from build123d import *

# Parameters (mm, degrees)
BOX013_W          = 14
BOX013_H          = 4.3
BOX013_DEPTH      = 10
CYLINDER021_R     = 28
CYLINDER021_DEPTH = 4
CYLINDER019_R     = 34
CYLINDER019_DEPTH = 13
CYLINDER020_R     = 25
CYLINDER020_DEPTH = 13
TUBE_R            = 34
TUBE_R_2          = 31
TUBE_DEPTH        = 23
EXTRUDE001_DEPTH  = 14
BOX012_W          = 10
BOX012_H          = 6
BOX012_DEPTH      = 10


with BuildPart() as cube013:
    # Box013 → Box013 (new body)
    with BuildSketch(Plane(origin=(64, 38.5, 50.5), x_dir=(1, 0, 0), z_dir=(0, 0, 1))):
        with Locations((7, 2.15)):
            Rectangle(BOX013_W, BOX013_H)
    extrude(amount=BOX013_DEPTH)


with BuildPart() as cylinder021:
    # Cylinder021 → Cylinder021 (new body)
    with BuildSketch(Plane(origin=(40, 40.65, 54), x_dir=(1, 0, 0), z_dir=(0, 0, 1))):
        Circle(CYLINDER021_R)
    extrude(amount=CYLINDER021_DEPTH)


with BuildPart() as cone:
    # Cone → Cone (revolve)
    with BuildSketch(Plane(origin=(40, 40.65, 53), x_dir=(1, 0, 0), z_dir=(0, -1, 0))):
        Polygon((0, 0), (26.5, 0), (31, 14), (0, 14), align=None)
    revolve(axis=Axis((40, 40.65, 53), (0, 0, 1)))


with BuildPart() as cylinder019:
    # Cylinder019 → Cylinder019 (new body)
    with BuildSketch(Plane(origin=(40, 40.65, 54), x_dir=(1, 0, 0), z_dir=(0, 0, 1))):
        Circle(CYLINDER019_R)
    extrude(amount=CYLINDER019_DEPTH)


with BuildPart() as cylinder020:
    # Cylinder020 → Cylinder020 (new body)
    with BuildSketch(Plane(origin=(40, 39.2, 54), x_dir=(1, 0, 0), z_dir=(0, 0, 1))):
        Circle(CYLINDER020_R)
    extrude(amount=CYLINDER020_DEPTH)


with BuildPart() as cut016:
    # Tube → Tube (new body)
    with BuildSketch(Plane(origin=(40, 40.65, 54), x_dir=(1, 0, 0), z_dir=(0, 0, 1))):
        Circle(TUBE_R)
        Circle(TUBE_R_2, mode=Mode.SUBTRACT)
    extrude(amount=TUBE_DEPTH)

    # Fusion010: union Cylinder019, Cylinder020
    add(cylinder019.part)
    add(cylinder020.part)

    # Cut015: cut Cone
    add(cone.part, mode=Mode.SUBTRACT)

    # Cut016: cut Cylinder021
    add(cylinder021.part, mode=Mode.SUBTRACT)


with BuildPart() as extrude001:
    # Sketch001 → Extrude001 (new body)
    with BuildSketch(Plane(origin=(0, 5, 65), x_dir=(1, 0, 0), z_dir=(0, 0, 1))):
        with BuildLine():
            ThreePointArc((16.057001, 41.301956), (16.937891, 38.759239), (19.112253, 37.173829))
            Line((19.112253, 37.173829), (24.78314, 35.869707))
            ThreePointArc((24.78314, 32.174329), (26.017604, 34.022018), (24.78314, 35.869707))
            Line((19.112253, 31.152458), (24.78314, 32.174329))
            ThreePointArc((19.112253, 31.152458), (16.911676, 29.555757), (16.032372, 26.983051))
            Line((15.813344, 26.918672), (16.032372, 26.983051))
            ThreePointArc((15.808908, 41.376289), (14.743203, 34.147153), (15.813344, 26.918672))
            Line((16.057001, 41.301956), (15.808908, 41.376289))
        make_face()
    extrude(amount=EXTRUDE001_DEPTH)


with BuildPart() as extrude001_1:
    # Extrude001 placement: moved
    add(extrude001.part.moved(Location((0, 0, 7))))


with BuildPart() as lid:
    # Box012 → Box012 (new body)
    with BuildSketch(Plane(origin=(7, 36.17, 76), x_dir=(1, 0, 0), z_dir=(0, 0, 1))):
        with Locations((5, 3)):
            Rectangle(BOX012_W, BOX012_H)
    extrude(amount=BOX012_DEPTH)

    # Fusion006: union Extrude001
    add(extrude001_1.part)


with BuildPart() as lid_1:
    # Fusion006 placement: moved
    add(lid.part.moved(Location((0, 1.5, -19))))

    # Fusion024: union Cut016
    add(cut016.part)

    # Cut017: cut Cube013
    add(cube013.part, mode=Mode.SUBTRACT)


solid = lid_1.part
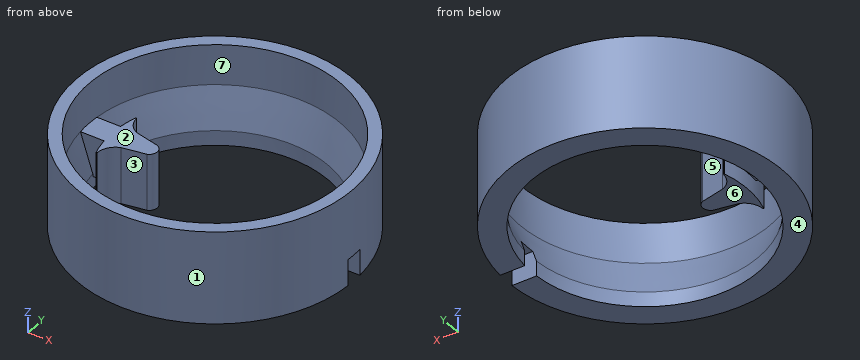
The listing builds one solid part. Answer for the finished solid, in the listing's coordinates (mm). Face numbers are marked on the shaded views. A direction names the side the tool comes from. Give positions to 0.01 mm unless a question says otherwise; leave off trailing zeros. Order: outer loops, then holes, each group sorted by start corner. A loop starts at its lowest first (then second) coordinate and runs counter-clockwise, first axis right, second up. Notation, with made-up numbers: (81, 29.5) -> (103, 29.5) arc R27 ccw to (103, 56.5) -> close; hole circle Ø1 at (70, -28.5). An arc over 180 degrees is marked (long way). Put each result on its own line as item: value.
Item 1: Given P1, Ø6.5, axis at x = 71.5, z = 56, coming from the +Y side; P2, Ø1, axis at x = 16, y = 34, coming from the +Z side; P3, Ø2, axis at x = 71.5, y = 40, coming from the -Z side; P4, Ø12, axis at x = 35, y = 21, coming from the -Z side (1 decimal), each flat-ended and moving along its own axis, determine where each tip first touches the part or whether it passes through.
Established:
P1: stops at y = 59.57
P2: stops at z = 67
P3: stops at z = 60.5
P4: passes through
Item 2: A cutting plane is placed at C-C on y = 40.65. Give the vertices of the cut face in (x, z), plus the area to 3 significant figures.
Established:
outline: (6, 54) -> (12, 54) -> (12, 57) -> (14.74, 57) -> (14.74, 53) -> (26.01, 53) -> (26.01, 67) -> (9, 67) -> (9, 77) -> (6, 77) -> close; (68.91, 60.5) -> (74, 60.5) -> (74, 77) -> (71, 77) -> (71, 67) -> close
area: 350 mm^2
Item 3: A cutting plane is placed at B-B on x = 40. Give the vertices of the cut face in (y, z), plus the area to 3 significant figures.
Established:
outline: (6.65, 54) -> (12.65, 54) -> (12.65, 57.67) -> (9.65, 67) -> (9.65, 77) -> (6.65, 77) -> close; (68.65, 54) -> (74.65, 54) -> (74.65, 77) -> (71.65, 77) -> (71.65, 67) -> (68.65, 57.67) -> close
area: 188 mm^2
Item 4: A cutting plane is placed at D-D on z = 59.5. Give the vertices of the cut face in (x, y) (3 decimals).
Established:
outline: (11.566, 37.67) -> (14.922, 37.67) arc R25 ccw to (15.813, 33.419) -> (16.032, 33.483) arc R4.5 cw to (19.112, 37.652) -> (24.783, 38.674) arc R2 ccw to (24.783, 42.37) -> (19.112, 43.674) arc R4.5 cw to (16.057, 47.802) -> (15.809, 47.876) arc R25 ccw to (14.926, 43.67) -> (11.571, 43.67) arc R28.589 cw to (68.508, 42.8) -> (73.932, 42.8) arc R34 ccw (long way) to (73.932, 38.5) -> (68.508, 38.5) arc R28.589 cw to start
Item 5: Straight lines are drawn through the part: line 1 (Y direction, x = 40, z = 71); line 2 (Y direction, x = 16, z = 61); line 3 (X direction, y = 44.5, z = 71.5). For each, find the intervals that lie inside material, in ascending order.
Established:
line 1: y = 6.65 to 9.65, 71.65 to 74.65
line 2: y = 16.57 to 24.24, 33.47 to 47.82, 57.06 to 64.73
line 3: x = 6.22 to 9.24, 70.76 to 73.78
Item 6: A cutting plane is placed at A-A on z = 55.25. Give the vertices of the cut face in (x, y) (3 decimals).
Established:
outline: (15.809, 47.876) arc R25 ccw to (15.813, 33.419) -> (16.032, 33.483) arc R4.5 cw to (19.112, 37.652) -> (24.783, 38.674) arc R2 ccw to (24.783, 42.37) -> (19.112, 43.674) arc R4.5 cw to (16.057, 47.802) -> close; (67.917, 38.5) arc R28 cw (long way) to (67.917, 42.8) -> (73.932, 42.8) arc R34 ccw (long way) to (73.932, 38.5) -> close
Item 7: For a pull along X with two mould halves and no side action, classify the marked faces 1, 2, 3 and 4 as released by +X, released by -X, zero draft, split by the parting line, or undercut.
Established:
face 1: split by the parting line
face 2: undercut
face 3: undercut
face 4: zero draft
Item 8: For the marked faces 5, 6 and 7, determine the directions among +Z, -Z, +X, -X, +Y, -Y from which every point of the face is accessible in a straight line to the end or side of a thin tool.
Established:
face 5: +Z, -Z
face 6: -Z, +X, -X, +Y, -Y
face 7: +Z
